Input: part model. Units: mm. Frame: model coordinates. A direction names the side the tool comes from. Coordinates: 2 decimals unless noted, no trailing zeros. Loops run counter-clockwise (first coordinate to the right, second up) from the corner with the lowest first, then second, coordinate; pieces in that order, holes last. Notation, with made-up numbers: (57, 73.25) -> (92, 73.25) arc R32 ccw to (92, 112.25) -> close; hole circle Ø11 at (60.25, 86.5). An arc over 180 degrees is marked (long way). Answer as a JSON object with one key per item and string values.
from build123d import *

# Parameters (mm, degrees)
FRAME_BODY_EXT_DEPTH                  = 6
FRAME_BODY_EXT_DEPTH_BACK             = 6
SKETCH6_R                             = 2.25
FRAME_BOLT_CUT_DEPTH                  = 26.13961018
SKETCH9_W                             = 12
SKETCH9_H                             = 12
CASE_BODY_EXT_DEPTH                   = 20
SKETCH10_R                            = 2.25
CASE_BOLT_CUT_DEPTH                   = 39.721912961
PRINT_PLANE_CUT_REACH                 = 31.479
SKETCH11_R                            = 4
CASE_COUNTERBORE_CUT_DEPTH            = 4
SKETCH7_R                             = 4
FRAME_COUNTERBORE_CUT_DEPTH           = 4
FRAME_COUNTERBORE_EXTENSION_CUT_DEPTH = 4
CASE_COUNTERBORE_EXTENSION_CUT_DEPTH  = 4
ROTATION_ONTO_PRINT_PLANE_ANGLE       = 45


with BuildPart() as part:
    # Sketch5 → Frame Body Ext (new, two sides: drawn at the far end of the back side and taken through both)
    with BuildSketch(Plane.ZY.offset(-FRAME_BODY_EXT_DEPTH_BACK)):
        Polygon((-20, 6), (-20, -11), (-23, -11), (-23, -14), (0, -14), (0, 6), align=None)
    extrude(amount=FRAME_BODY_EXT_DEPTH + FRAME_BODY_EXT_DEPTH_BACK)

    # Sketch6 → Frame Bolt Cut (cut, through all)
    with BuildSketch(Plane(origin=(0, 0, -20), x_dir=(-1, 0, 0), z_dir=(0, 0, -1))):
        Circle(SKETCH6_R)
    extrude(amount=-FRAME_BOLT_CUT_DEPTH, mode=Mode.SUBTRACT)

    # Sketch9 → Case Body Ext (add)
    with BuildSketch(Plane(origin=(12, 7.071067812, 3.571067812), x_dir=(-1, 0, 0), z_dir=(0, -0.7071067811865486, -0.7071067811865465))):
        Rectangle(SKETCH9_W, SKETCH9_H)
    extrude(amount=CASE_BODY_EXT_DEPTH)

    # Sketch10 → Case Bolt Cut (cut, through all)
    with BuildSketch(Plane(origin=(0, 5.321067812, 5.321067812), x_dir=(1, 0, 0), z_dir=(0, 0.7071067811865487, 0.7071067811865465))):
        with Locations(Location((12, 2.474873734, 0), (0, 0, 270))):
            Circle(SKETCH10_R)
    extrude(amount=-CASE_BOLT_CUT_DEPTH, mode=Mode.SUBTRACT)

    # Sketch14 → Print Plane Cut (cut, up to next)
    with BuildSketch(Plane(origin=(6, 0, 0), x_dir=(0, 0, -1), z_dir=(1, 0, 0)), mode=Mode.PRIVATE) as print_plane_cut_sk1:
        Polygon((0, -4.985281374), (9.014718626, -14), (0, -14), align=None)
    print_plane_cut_tool1 = extrude(print_plane_cut_sk1.sketch, amount=-PRINT_PLANE_CUT_REACH, mode=Mode.PRIVATE) & part.part
    add(print_plane_cut_tool1.solids().sort_by_distance((6, -10.995094, -3.004906))[0], mode=Mode.SUBTRACT)

    # Sketch11 → Case Counterbore Cut (cut)
    with BuildSketch(Plane(origin=(0, -8.821067812, -8.821067812), x_dir=(1, 0, 0), z_dir=(0, -0.7071067811865487, -0.7071067811865465))):
        with Locations(Location((12, -2.474873734, 0), (0, 0, 270))):
            Circle(SKETCH11_R)
    extrude(amount=-CASE_COUNTERBORE_CUT_DEPTH, mode=Mode.SUBTRACT)

    # Sketch7 → Frame Counterbore Cut (cut)
    with BuildSketch(Plane.XY):
        Circle(SKETCH7_R)
    extrude(amount=-FRAME_COUNTERBORE_CUT_DEPTH, mode=Mode.SUBTRACT)

    # Sketch15 → Frame Counterbore Extension Cut (cut)
    with BuildSketch(Plane.XY):
        with BuildLine():
            Line((-4, 0), (-4, 6))
            Line((-4, 6), (4, 6))
            Line((4, 6), (4, 0))
            ThreePointArc((4, 0), (0, 4), (-4, 0))
        make_face()
    extrude(amount=-FRAME_COUNTERBORE_EXTENSION_CUT_DEPTH, mode=Mode.SUBTRACT)

    # Sketch16 → Case Counterbore Extension Cut (cut)
    with BuildSketch(Plane(origin=(0, -8.821067812, -8.821067812), x_dir=(1, 0, 0), z_dir=(0, -0.7071067811865486, -0.7071067811865465))):
        with BuildLine():
            Line((16, -8.474873734), (16, -2.474873734))
            ThreePointArc((16, -2.474873734), (12, -6.474873734), (8, -2.474873734))
            Line((8, -2.474873734), (8, -8.474873734))
            Line((8, -8.474873734), (16, -8.474873734))
        make_face()
    extrude(amount=-CASE_COUNTERBORE_EXTENSION_CUT_DEPTH, mode=Mode.SUBTRACT)


with BuildPart() as part_1:
    # Rotation onto Print Plane: read off the stored shape, not the designer's step
    # Rotation onto Print Plane: moved
    add(part.part.moved(Location((0, 6.8388348, 1.8535534))).rotate(Axis((0, 0, 0), (1, 0, 0)), ROTATION_ONTO_PRINT_PLANE_ANGLE))


solid = part_1.part
1. Line query: line 1 along X through (y, z) = (6, 6.5); line 2 along X through (y, z) = (15.75, 2); line 3 along Y through (x, z) = (1.5, -0.5). Output: solid intervals per line, ascending.
Reply:
{"line 1": "x = -6 to -4, 4 to 9.75, 14.25 to 18", "line 2": "x = -6 to 6", "line 3": "y = 0 to 7.8, 12.54 to 18.66"}
2. Mould query, pull axis Y, two halves, no side actions, for faces 6 (the face through (0.084, 10.965, -18.941)), 7 (the face through (2.75, 1.24, 3.86)), 8 (the face through (4, 7, 7)). Classes: pulls with the +Y half, pulls with the -Y half, needs draft (parallel to the pull), parting line crosses it, or undercut.
Reply:
{"face 6": "pulls with the +Y half", "face 7": "pulls with the -Y half", "face 8": "undercut"}
3. Section query C-C (y = 11). Count the separate pieces of the cut face and the enclosed holes in it, plus the area to 3 significant figures.
Reply:
{"separate pieces": "2", "enclosed holes": "1", "area": "472 mm2"}
4. Pin query (flat end, axial travel): P1, Ø1.5, axis at x = 9, y = 10.5, coming from the -Z side; P2, Ø1.5, axis at x = 7.5, z = -14, coming from the -Y side; P3, Ø1, axis at y = 5.5, z = 9, coming from the -X side; P4, Ø6.5, axis at x = 13, y = 5, coming from the -Z side. Return the tip coordinate at first contact, or that it passes through.
Reply:
{"P1": "stops at z = -2.33", "P2": "passes through", "P3": "stops at x = 6", "P4": "stops at z = -6.33"}
5. Section query B-B (x = 0.5). Return loops of the section in (y, z).
Reply:
{"outline": "(0, -10.13) -> (9.89, -20.02) -> (12.01, -17.9) -> (9.89, -15.77) -> (16.12, -9.55) -> (4.8, 1.77) -> (3.55, 0.51) -> (0.72, 3.34) -> (0, 2.62) -> close; (7.9, 4.87) -> (19.22, -6.44) -> (21.91, -3.75) -> (10.6, 7.56) -> close"}
6. Section query A-A (x = 12). Return loops of the section in (y, z).
Reply:
{"outline": "(0, -6.33) -> (2, -6.33) -> (2, -2.33) -> (3.75, -2.33) -> (3.75, 13.67) -> (0, 13.67) -> close; (8.25, -2.33) -> (12, -2.33) -> (12, 13.67) -> (8.25, 13.67) -> close"}
7. Access query for faces 1 (the face through (13.42, 2.08, -6.328)), 2 (the face through (12, 9, -2.328)), 3 (the face through (0.084, 10.935, -16.82)), 4 (the face through (0.056, 8.682, 5.646)), 5 (the face through (12, 12, 6)). Directions: +Z, -Z, +X, -X, +Y, -Y. A direction counts if a zero-diameter tool reaches every point of the face in a straight line with its end or side. Return the directions, or none.
Reply:
{"face 1": "-Z, +X, +Y, -Y", "face 2": "-Z, +Y", "face 3": "+X, -X, +Y", "face 4": "+Z", "face 5": "+Z, -Z, +X, +Y"}
